Check sheet for the drawn part. Datum: minimum x, y, z corner. Units: mm. A direction names the side the tool comes from. Round coordinates to 2 decimals unless told otherwise and drop trailing zeros. Write each loop counter-clockwise with the first axis right and the second up, starting at its lowest first coordinate (ties: lowest second). Pieces come first, ordered by that corner, then holes. Notation, with made-up numbers: M 36.25,47.5 L 41.25,47.5 A16 ccw 41.25,69.5 Z; hole C 0,18.5 d4. An arc over 180 degrees is marked long. One line per item, written item: value.
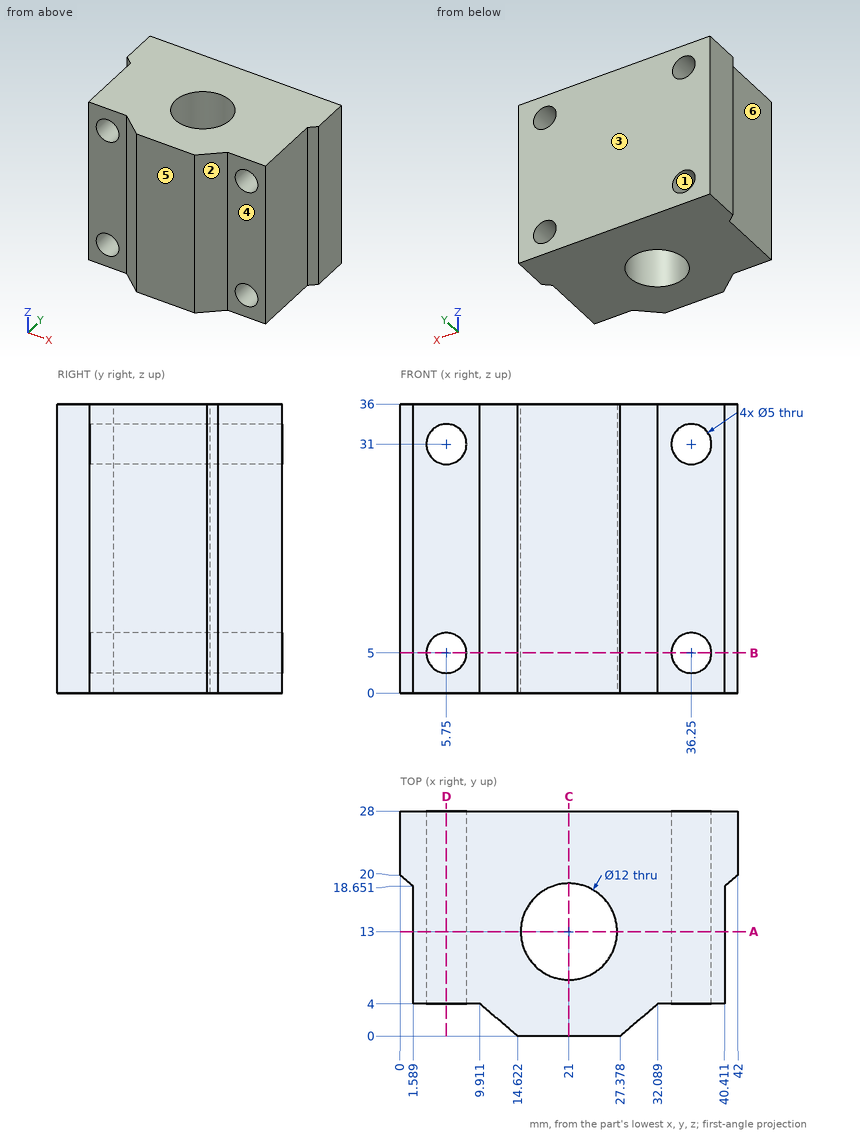
Q1. Sectioned sample at B-B on z = 5. Enter the section's corners in (x, y).
Completed:
outline: M 0,20 L 1.59,18.65 L 1.59,4 L 3.25,4 L 3.25,28 L 0,28 Z; M 8.25,4 L 9.91,4 L 14.62,0 L 27.38,0 L 32.09,4 L 33.75,4 L 33.75,28 L 8.25,28 Z; M 38.75,4 L 40.41,4 L 40.41,18.65 L 42,20 L 42,28 L 38.75,28 Z; hole C 21,13 d12
Q2. Sectioned sample at C-C on x = 21. Enter the section's corners in (y, z).
Completed:
outline: M 0,0 L 7,0 L 7,36 L 0,36 Z; M 19,0 L 28,0 L 28,36 L 19,36 Z
Q3. Scan lines: line 1 (Z direction, x = 5.75, y = 9); line 2 (Z direction, x = 37, y = 8.25) (1 decimal); line 3 (X direction, y = 20.75, z = 7). Record each from-to range of solid material in increasing order. Write a range as [from, to].
Completed:
line 1: [0, 2.5], [7.5, 28.5], [33.5, 36]
line 2: [0, 2.6], [7.4, 28.6], [33.4, 36]
line 3: [0, 4.25], [7.25, 34.75], [37.75, 42]
Q4. Access from +Z, -Z, +X, -X, +Y, -Y to the whole of each face (thin tool, end or side, straight path). Record for the marked faces 4, 5 and 6.
Completed:
face 4: +Z, -Z, +X, -Y
face 5: +Z, -Z, +X, -X, -Y
face 6: +Z, -Z, -X, -Y
Q5. Depth check by flat-ended pin: P1, Ø6.5, axis at x = 7.5, z = 13, coming from the -Y side; P2, Ø12, axis at x = 27, z = 13, coming from the -Y side; P3, Ø4, axis at y = 3.5, z = 26.5, coming from the -X side; P4, Ø4.5, axis at x = 36.25, z = 31, coming from the -Y side. Enter the tip coordinate at first touch or a pass-through.
Completed:
P1: y = 3.29
P2: y = 0
P3: x = 1.59
P4: through
Q6. Draft check along X on the marked faces 1, 2 and 3. Enter one of: pulls with the +X half, pulls with the -X half, needs draft (parallel to the pull), parting line crosses it, or undercut.
Completed:
face 1: undercut
face 2: pulls with the +X half
face 3: needs draft
Q7. Sectioned sample at A-A on y = 13. Enter the section's corners in (x, z), and give its area (3 significant figures).
Completed:
outline: M 1.59,0 L 15,0 L 15,36 L 1.59,36 Z; M 27,0 L 40.41,0 L 40.41,36 L 27,36 Z; hole C 5.75,5 d5; hole C 5.75,31 d5; hole C 36.25,5 d5; hole C 36.25,31 d5
area: 887 mm^2
Q8. Sectioned sample at D-D on x = 5.75. Enter the section's corners in (y, z), and give its area (3 significant figures).
Completed:
outline: M 4,0 L 28,0 L 28,2.5 L 4,2.5 Z; M 4,7.5 L 28,7.5 L 28,28.5 L 4,28.5 Z; M 4,33.5 L 28,33.5 L 28,36 L 4,36 Z
area: 624 mm^2
